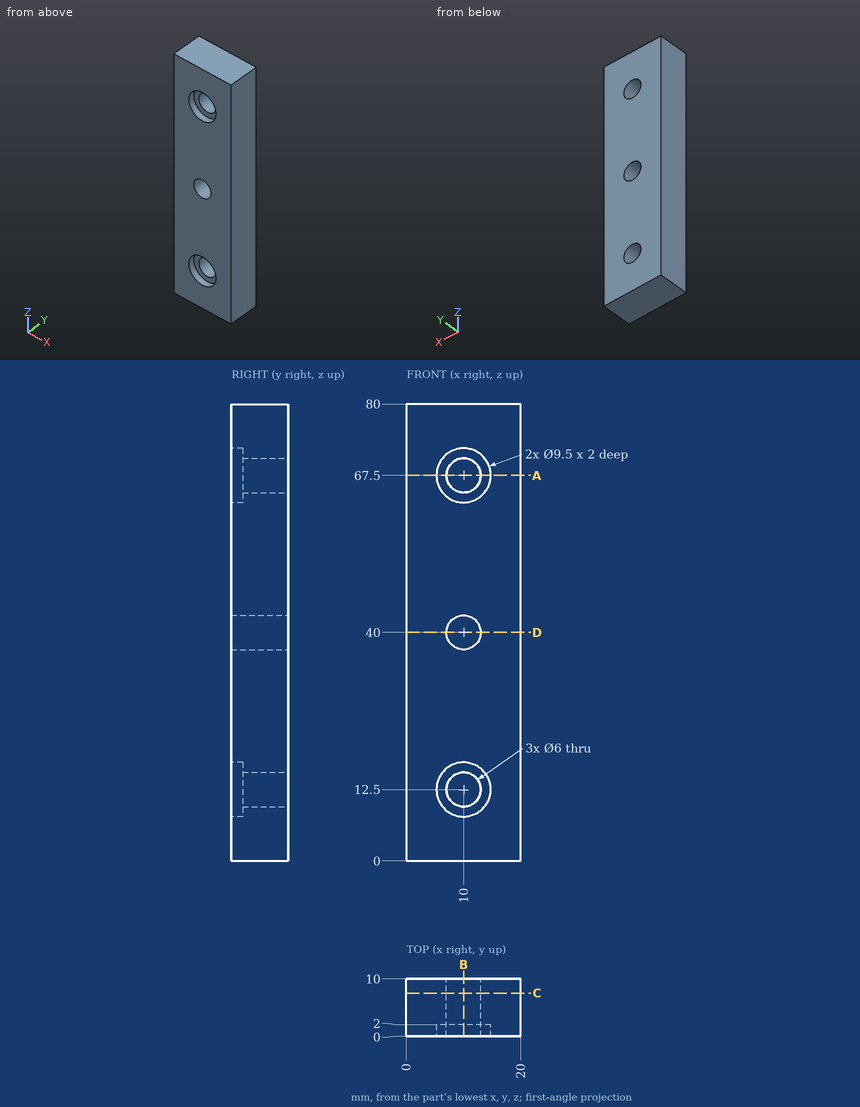
Answer from the drawing. Dimensions are ordinates in mm from the lowest x, y and z of the part. Give positions to 0.01 mm unless a question says otherwise; leave off trailing zeros. Order: outer loops, then holes, each group sorted by start corner. A loop starts at its lowest first (then second) coordinate and runs counter-clockwise, first axis right, second up. Notation, with made-up numbers: (77.25, 26.5) - (88.25, 26.5) arc R25 ccw to (88.25, 60.5) - close; hole circle Ø2 at (-38.75, 53.5). An arc over 180 degrees is marked (long way). One line per item, written item: value. Start each with the question number.
1. Section D-D, the plane z = 40 is taken. Write down the section's boundary in (x, y).
2. Consider line 1 (Z direction, x = 10, y = 1.1); line 2 (Z direction, x = 10, y = 7.5); line 3 (X direction, y = 7, z = 67.5). Determine where each line is inside the solid, lowest interval first.
3. Section B-B, the plane x = 10 is taken. Write down the section's boundary in (y, z), then the cut area to 3 significant figures.
4. Section C-C, the plane y = 7.5 is taken. Write down the section's boundary in (x, z).
5. Section A-A, the plane z = 67.5 is taken. Write down the section's boundary in (x, y).
Filled sheet:
1. outline: (0, 0) - (7, 0) - (7, 10) - (0, 10) - close; (13, 0) - (20, 0) - (20, 10) - (13, 10) - close
2. line 1: 0 to 7.75, 17.25 to 37, 43 to 62.75, 72.25 to 80
2. line 2: 0 to 9.5, 15.5 to 37, 43 to 64.5, 70.5 to 80
2. line 3: 0 to 7, 13 to 20
3. outline: (0, 0) - (10, 0) - (10, 9.5) - (2, 9.5) - (2, 7.75) - (0, 7.75) - close; (0, 17.25) - (2, 17.25) - (2, 15.5) - (10, 15.5) - (10, 37) - (0, 37) - close; (0, 43) - (10, 43) - (10, 64.5) - (2, 64.5) - (2, 62.75) - (0, 62.75) - close; (0, 72.25) - (2, 72.25) - (2, 70.5) - (10, 70.5) - (10, 80) - (0, 80) - close
3. area: 606 mm²
4. outline: (0, 0) - (20, 0) - (20, 80) - (0, 80) - close; hole circle Ø6 at (10, 12.5); hole circle Ø6 at (10, 40); hole circle Ø6 at (10, 67.5)
5. outline: (0, 0) - (5.25, 0) - (5.25, 2) - (7, 2) - (7, 10) - (0, 10) - close; (13, 2) - (14.75, 2) - (14.75, 0) - (20, 0) - (20, 10) - (13, 10) - close
